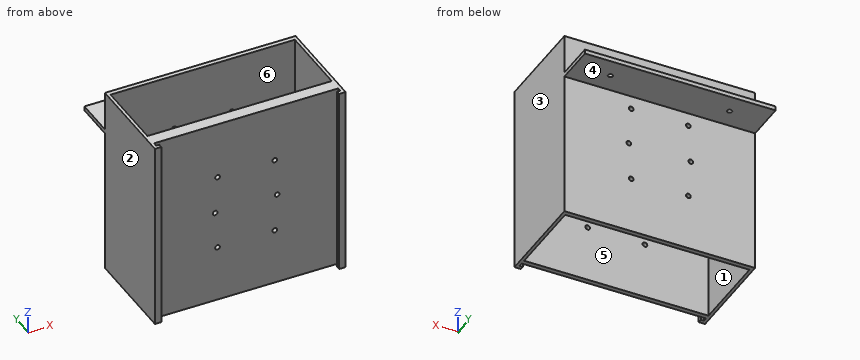
```python
from build123d import *

# Parameters (mm, degrees)
SKETCH_2_W          = 120
SKETCH_2_H          = 120
EXTRUDE_1_DEPTH     = 3
SKETCH_5_W          = 2
SKETCH_5_H          = 120
EXTRUDE_3_DEPTH     = 50
SKETCH_6_W          = 120
SKETCH_6_H          = 120
EXTRUDE_4_DEPTH     = 3
SKETCH_7_W          = 116
SKETCH_7_H          = 1.5
EXTRUDE_5_DEPTH     = 5
SKETCH_9_W          = 120
SKETCH_9_H          = 2.735218368
EXTRUDE_6_DEPTH     = 25
SKETCH_11_R         = 1.5
CUT_EXTRUDE_1_DEPTH = 58
SKETCH_10_R         = 1.5
CUT_EXTRUDE_2_DEPTH = 3
SKETCH_13_W         = 4
SKETCH_13_H         = 120
EXTRUDE_10_DEPTH    = 5
SKETCH_14_W         = 2
SKETCH_14_H         = 2.5
CUT_EXTRUDE_3_DEPTH = 120


with BuildPart() as part:
    # 草图2 → 凸台-拉伸1 (new body)
    with BuildSketch(Plane(origin=(0, 0, 0), x_dir=(1, 0, 0), z_dir=(0, 1, 0))):
        with Locations((60, -60)):
            Rectangle(SKETCH_2_W, SKETCH_2_H)
    extrude(amount=EXTRUDE_1_DEPTH)

    # 草图5 → 凸台-拉伸3 (add)
    with BuildSketch(Plane(origin=(0, 3, 0), x_dir=(1, 0, 0), z_dir=(0, 1, 0))):
        with Locations((1, -60)):
            Rectangle(SKETCH_5_W, SKETCH_5_H)
        with Locations((119, -60)):
            Rectangle(SKETCH_5_W, SKETCH_5_H)
    extrude(amount=EXTRUDE_3_DEPTH)

    # 草图6 → 凸台-拉伸4 (add)
    with BuildSketch(Plane(origin=(0, 53, 0), x_dir=(1, 0, 0), z_dir=(0, 1, 0))):
        with Locations((60, -60)):
            Rectangle(SKETCH_6_W, SKETCH_6_H)
    extrude(amount=EXTRUDE_4_DEPTH)

    # 草图7 → 凸台-拉伸5 (add)
    with BuildSketch(Plane(origin=(0, 3, 0), x_dir=(1, 0, 0), z_dir=(0, 1, 0))):
        with Locations((60, -119.25)):
            Rectangle(SKETCH_7_W, SKETCH_7_H)
    extrude(amount=EXTRUDE_5_DEPTH)

    # 草图9 → 凸台-拉伸6 (add)
    with BuildSketch(Plane(origin=(0, 56, 0), x_dir=(1, 0, 0), z_dir=(0, 1, 0))):
        with Locations((60, -93.632390816)):
            Rectangle(SKETCH_9_W, SKETCH_9_H)
    extrude(amount=EXTRUDE_6_DEPTH)

    # 草图11 → 切除-拉伸1 (cut)
    with BuildSketch(Plane(origin=(0, 56, 0), x_dir=(1, 0, 0), z_dir=(0, 1, 0))):
        with Locations(Location((42, -35.764781632, 0), (0, 0, 270))):
            Circle(SKETCH_11_R)
        with Locations(Location((40.5, -59.764781632, 0), (0, 0, 270))):
            Circle(SKETCH_11_R)
        with Locations(Location((42, -83.764781632, 0), (0, 0, 270))):
            Circle(SKETCH_11_R)
        with Locations(Location((79.5, -59.764781632, 0), (0, 0, 270))):
            Circle(SKETCH_11_R)
        with Locations(Location((78, -83.764781632, 0), (0, 0, 270))):
            Circle(SKETCH_11_R)
        with Locations(Location((78, -35.764781632, 0), (0, 0, 270))):
            Circle(SKETCH_11_R)
    extrude(amount=-CUT_EXTRUDE_1_DEPTH, mode=Mode.SUBTRACT)

    # 草图10 → 切除-拉伸2 (cut)
    with BuildSketch(Plane.XY.offset(95)):
        with Locations((22.5, 68.5)):
            Circle(SKETCH_10_R)
        with Locations((97.5, 68.5)):
            Circle(SKETCH_10_R)
    extrude(amount=-CUT_EXTRUDE_2_DEPTH, mode=Mode.SUBTRACT)

    # 草图13 → 凸台-拉伸10 (add)
    with BuildSketch(Plane(origin=(0, 0, 0), x_dir=(-1, 0, 0), z_dir=(0, -1, 0))):
        with Locations((-2, -60)):
            Rectangle(SKETCH_13_W, SKETCH_13_H)
        with Locations((-118, -60)):
            Rectangle(SKETCH_13_W, SKETCH_13_H)
    extrude(amount=EXTRUDE_10_DEPTH)

    # 草图14 → 切除-拉伸3 (cut)
    with BuildSketch(Plane(origin=(0, 0, 0), x_dir=(-1, 0, 0), z_dir=(0, 0, -1))):
        with Locations((-117, -1.25)):
            Rectangle(SKETCH_14_W, SKETCH_14_H)
        with Locations((-3, -1.25)):
            Rectangle(SKETCH_14_W, SKETCH_14_H)
    extrude(amount=-CUT_EXTRUDE_3_DEPTH, mode=Mode.SUBTRACT)


solid = part.part
```
Here's how the part is built. I have some questions about the finished solid (model axes, mm). Face numbers are marked on the shaded views. A direction names the side the tool comes from. Round coordinates to 2 decimals unless told otherwise and drop trailing zeros. Loops run counter-clockwise (first coordinate to the right, second up) from the corner with the lowest first, then second, coordinate; pieces in that order, holes last.
1. Suppose I cut it at A-A, the plane x = 27. Please give me the cut outline in (y, z).
Answers:
outline: (0, 0) - (3, 0) - (3, 118.5) - (8, 118.5) - (8, 120) - (0, 120) - close; (53, 0) - (56, 0) - (56, 92.26) - (81, 92.26) - (81, 95) - (56, 95) - (56, 120) - (53, 120) - close
2. Will these pins go through, and if not, where does the flat tip stop? pin 1 (4 mm diameter, centred on x = 61, z = 72, fed in from +Y); pin 2 (4 mm diameter, centred on x = 59, z = 77, fed in from -Y); pin 3 (4 mm diameter, centred on x = 22.5, y = 68.5, fed in from +Z).
Answers:
pin 1: stops at y = 56
pin 2: stops at y = 0
pin 3: stops at z = 95
3. If I drill on probe 1 along Y at (x, z) = (22.5, 92.85); probe 2 along Y at (x, z) = (6, 30); probe 3 along X at (y, z) = (51, 61), over which ranges is the centre line in solid material (lowest first)?
Answers:
probe 1: y = 0 to 3, 53 to 67, 70 to 81
probe 2: y = 0 to 3, 53 to 56
probe 3: x = 0 to 2, 118 to 120
4. Suppose I cut it at B-B, the plane z = 112. Please give me the cut outline in (x, y).
Answers:
outline: (0, -5) - (4, -5) - (4, -2.5) - (2, -2.5) - (2, 0) - (118, 0) - (118, -2.5) - (116, -2.5) - (116, -5) - (120, -5) - (120, 56) - (0, 56) - close; hole (2, 3) - (118, 3) - (118, 53) - (2, 53) - close
5. For the marked faces 4, 5 and 6, which set-ups out of +Z, -Z, +X, -X, +Y, -Y let a thin tool reach every point of the face, with its end or its side?
Answers:
face 4: -Z, +X, -X, +Y
face 5: -Z
face 6: +Z, -Z
6. Suppose I cut it at C-C, the plane y = 25. Please give me the cut outline in (x, z).
Answers:
outline: (0, 0) - (2, 0) - (2, 120) - (0, 120) - close; (118, 0) - (120, 0) - (120, 120) - (118, 120) - close
7. Thinking about a two-plate mould opening in X: for the marked faces 1, 2 and 3, which applies, released by +X, released by -X, zero draft, split by the parting line, or undercut?
Answers:
face 1: undercut
face 2: released by -X
face 3: released by +X
